```python
from build123d import *

# Parameters (mm, degrees)
F0_W        = 200
F0_H        = 10
F1_DEPTH    = 14.9
F2_W        = 10
F2_H        = 2.9
F3_DEPTH    = 10
F4_R        = 1.5
F5_DEPTH    = 14.9
F6_T1_DEPTH = 218.4999999506
F6_T3_DEPTH = 218.4999999928


# Not quite as in the source:
# - a fillet or chamfer that OpenCascade refuses, or shapes differently, is made with other operations: its cross-section is extruded or revolved along the edge and cut away or added


with BuildPart() as f1:
    # F0 (on Front) → F1 (new body)
    with BuildSketch(Plane.XZ):
        Rectangle(F0_W, F0_H)
    extrude(amount=F1_DEPTH)

    # F2 (on face) → F3 (join)
    with BuildSketch(Plane.XY.offset(5)):
        with Locations((-105, -13.45)):
            Rectangle(F2_W, F2_H)
        with Locations((-105, -7.45)):
            Rectangle(F2_W, F2_H)
        with Locations((-105, -1.45)):
            Rectangle(F2_W, F2_H)
        with Locations((105, -13.45)):
            Rectangle(F2_W, F2_H)
        with Locations((105, -7.45)):
            Rectangle(F2_W, F2_H)
        with Locations((105, -1.45)):
            Rectangle(F2_W, F2_H)
    extrude(amount=-F3_DEPTH)

    # F4 (on face) → F5 (cut)
    with BuildSketch(Plane(origin=(0, 0, 0), x_dir=(-1, 0, 0), z_dir=(0, 1, 0))):
        with BuildLine():
            ThreePointArc((-110, 0), (-108.5355339059, 3.5355339059), (-105, 5))
            Line((-105, 5), (-110, 5))
            Line((-110, 5), (-110, 0))
        make_face()
        with BuildLine():
            Line((-110, -5), (-105, -5))
            ThreePointArc((-105, -5), (-108.5355339059, -3.5355339059), (-110, 0))
            Line((-110, 0), (-110, -5))
        make_face()
        with Locations((-105, 0)):
            Circle(F4_R)
        with BuildLine():
            ThreePointArc((110, 0), (108.5355338885, -3.5355339234), (104.9999999506, -5))
            Line((104.9999999506, -5), (110, -5))
            Line((110, -5), (110, 0))
        make_face()
        with BuildLine():
            Line((110, 5), (104.9999999928, 5))
            ThreePointArc((104.9999999928, 5), (108.5355339034, 3.5355339085), (110, 0))
            Line((110, 0), (110, 5))
        make_face()
        with Locations((105, 0)):
            Circle(F4_R)
    extrude(amount=-F5_DEPTH, mode=Mode.SUBTRACT)

    # F6: fillet of radius 1 on 4 edges, made by hand

    # F6_s2 → F6_t1 (cut)
    with BuildSketch(Plane.YZ.offset(-109.2499999506)):
        with BuildLine():
            ThreePointArc((-1, -5), (-0.2928932188, -4.7071067812), (0, -4))
            Line((0, -4), (0, -5))
            Line((0, -5), (-1, -5))
        make_face()
        with BuildLine():
            ThreePointArc((-13.9, -5), (-14.6071067812, -4.7071067812), (-14.9, -4))
            Line((-14.9, -4), (-14.9, -5))
            Line((-14.9, -5), (-13.9, -5))
        make_face()
    extrude(amount=F6_T1_DEPTH, mode=Mode.SUBTRACT)

    # F6_s4 → F6_t3 (cut)
    with BuildSketch(Plane.YZ.offset(-109.2499999928)):
        with BuildLine():
            ThreePointArc((-1, 5), (-0.2928932188, 4.7071067812), (0, 4))
            Line((0, 4), (0, 5))
            Line((0, 5), (-1, 5))
        make_face()
        with BuildLine():
            ThreePointArc((-13.9, 5), (-14.6071067812, 4.7071067812), (-14.9, 4))
            Line((-14.9, 4), (-14.9, 5))
            Line((-14.9, 5), (-13.9, 5))
        make_face()
    extrude(amount=F6_T3_DEPTH, mode=Mode.SUBTRACT)


solid = f1.part
```
Can you work these out from the model? Positions are in its coordinate system, mm. A direction names the side the tool comes from. Coordinates: 2 decimals unless noted, no trailing zeros. Put each result on its own line as item: value. Start each with the question number.
(1) Will these pins go through, and if not, where does the flat tip stop? pin 1 Ø2.5 at (x, z) = (105, 0) entering from +Y; pin 2 Ø3.5 at (y, z) = (-4.5, 1.5) entering from +X; pin 3 Ø0.9 at (y, z) = (-5, 1) entering from -X.
(2) Which directions (+Z, -Z, +X, -X, +Y, -Y) give clear straight access to the entire face, cutting with the end or side of a thin tool? Please do faces 4 (the face through (-103, -2.9, 0)), 5 (the face through (-1, -7, -5)), 6 (the face through (103.8, -2.9, 1.2)).
(3) We'd pull the mould along Y, two halves only. Please class faces 1 (the face through (-2, -14.9, 0)), 2 (the face through (-103, -12, 0)), 3 (the face through (-1, -7, 5)): +Y half, -Y half, draft (parallel to the pull), parting line (faces both ways), or undercut.
(4) I need wall thicknesses on probe 1 along Z at (x, y) = (105, -2.15); probe 2 along X at (y, z) = (-4.25, 0.5); probe 3 along X at (y, z) = (-2.75, 4). Which ranges of each line are inside material? Lowest first, please.
Worked answers:
1. pin 1: passes through
1. pin 2: stops at x = 109.96
1. pin 3: stops at x = -100
2. face 4: +Z, -Z, -X
2. face 5: -Z, +X, -X, +Y, -Y
2. face 6: +Z, -Z, +X
3. face 1: -Y half
3. face 2: undercut
3. face 3: draft
4. probe 1: z = -5 to -1.5, 1.5 to 5
4. probe 2: x = -100 to 100
4. probe 3: x = -108 to 108
